Part model, mm, in its own coordinate system. Face numbers are marked on the shaded views. A direction names the side the tool comes from. Give positions to 0.01 mm unless a question says otherwise; leave off trailing zeros. Loops run counter-clockwise (first coordinate to the right, second up) from the corner with the lowest first, then second, coordinate; pieces in that order, holes last. Notation, with made-up numbers: (5, -32) -> (21, -32) arc R26 ccw to (21, -4) -> close; hole circle Ø1 at (67, 83.5). An arc over 180 degrees is marked (long way). One line per question, with ' | ' between items.
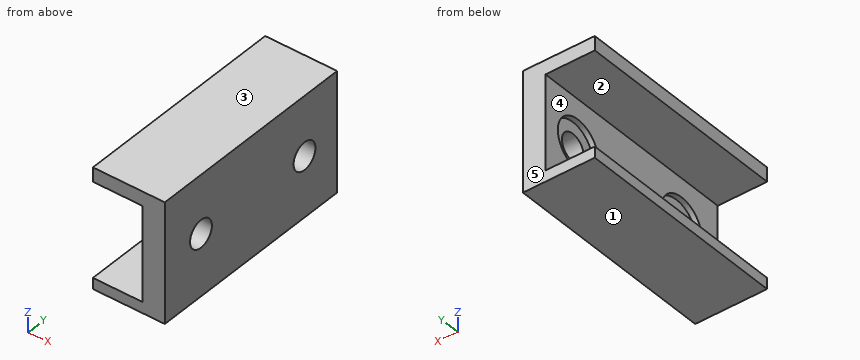
```python
from build123d import *

# Parameters (mm, degrees)
F0_W     = 36
F0_H     = 20
F1_DEPTH = 12
F2_W     = 43.75383
F2_H     = 15.8
F3_DEPTH = 8.24
F4_R     = 2.285
F5_DEPTH = 34.9
F6_R     = 4.215
F7_DEPTH = 9.1


with BuildPart() as f1:
    # F0 (on Right) → F1 (new body)
    with BuildSketch(Plane.YZ):
        with Locations((-48.512831, 15.170117)):
            Rectangle(F0_W, F0_H)
    extrude(amount=F1_DEPTH)

    # F2 (on Right) → F3 (cut)
    with BuildSketch(Plane.YZ):
        with Locations((-48.435772, 14.905577)):
            Rectangle(F2_W, F2_H)
    extrude(amount=F3_DEPTH, mode=Mode.SUBTRACT)

    # F4 (on Right) → F5 (cut)
    with BuildSketch(Plane.YZ):
        with Locations((-37.319533, 15.256222)):
            Circle(F4_R)
        with Locations((-58.956481, 15.463678)):
            Circle(F4_R)
    extrude(amount=F5_DEPTH, mode=Mode.SUBTRACT)

    # F6 (on Right) → F7 (cut)
    with BuildSketch(Plane.YZ):
        with Locations((-37.319533, 15.256222)):
            Circle(F6_R)
        with Locations((-58.956481, 15.463678)):
            Circle(F6_R)
    extrude(amount=F7_DEPTH, mode=Mode.SUBTRACT)


solid = f1.part
```
1) Saw through at D-D (y = -36.5). Give the cut face in (x, z), and give its area (3 significant figures).
Found:
outline: (0, 5.17) -> (12, 5.17) -> (12, 13.12) -> (9.1, 13.12) -> (9.1, 11.12) -> (8.24, 11.12) -> (8.24, 7.01) -> (0, 7.01) -> close; (0, 22.81) -> (8.24, 22.81) -> (8.24, 19.39) -> (9.1, 19.39) -> (9.1, 17.39) -> (12, 17.39) -> (12, 25.17) -> (0, 25.17) -> close | area: 90.3 mm2
2) Saw through at A-A (x = 7.25). Give the cut face in (y, z), and give its area (3 significant figures).
Found:
outline: (-66.51, 5.17) -> (-30.51, 5.17) -> (-30.51, 7.01) -> (-66.51, 7.01) -> close; (-66.51, 22.81) -> (-30.51, 22.81) -> (-30.51, 25.17) -> (-66.51, 25.17) -> close | area: 151 mm2
3) Drill centre lines: line 1 (Z direction, x = 2.25, y = -44); line 2 (Y direction, x = 11.75, z = 13.5); line 3 (Y direction, x = 11.25, z = 15.5). Where is each one in solid material? Low to high.
Found:
line 1: 5.17 to 7.01, 22.81 to 25.17 | line 2: -66.51 to -60.12, -57.79 to -38.78, -35.86 to -30.51 | line 3: -66.51 to -61.24, -56.67 to -39.59, -35.05 to -30.51
4) Saw through at C-C (z = 16.5). Give the cut face in (x, y), and give its area (3 significant figures).
Found:
outline: (8.24, -66.51) -> (12, -66.51) -> (12, -60.99) -> (9.1, -60.99) -> (9.1, -63.04) -> (8.24, -63.04) -> close; (8.24, -54.87) -> (9.1, -54.87) -> (9.1, -56.92) -> (12, -56.92) -> (12, -39.24) -> (9.1, -39.24) -> (9.1, -41.35) -> (8.24, -41.35) -> close; (8.24, -33.29) -> (9.1, -33.29) -> (9.1, -35.4) -> (12, -35.4) -> (12, -30.51) -> (8.24, -30.51) -> close | area: 98.5 mm2
5) Saw through at B-B (y = -51.5). Give the cut face in (x, z).
Found:
outline: (0, 5.17) -> (12, 5.17) -> (12, 25.17) -> (0, 25.17) -> (0, 22.81) -> (8.24, 22.81) -> (8.24, 7.01) -> (0, 7.01) -> close
6) Pull direction Z, two halves, no side cores. Call the marked faces 3, 4 and 5: pulls with the +Z half, pulls with the -Z half, needs draft (parallel to the pull), parting line crosses it, or undercut.
Found:
face 3: pulls with the +Z half | face 4: undercut | face 5: needs draft
7) Tool access for the marked faces 1 and 2: list every direction of +Z, -Z, +X, -X, +Y, -Y with a clear straight run to the whole face (end or side of a thin tool).
Found:
face 1: -Z, +X, -X, +Y, -Y | face 2: -X, +Y, -Y
8) Pin check, flat tips, straight feed: P1, Ø1, axis at y = -59, z = 19.5, coming from the -X side; P2, Ø6.5, axis at y = -59, z = 15, coming from the -X side. Stop position of each tip, or through.
Found:
P1: x = 8.24 | P2: x = 9.1
